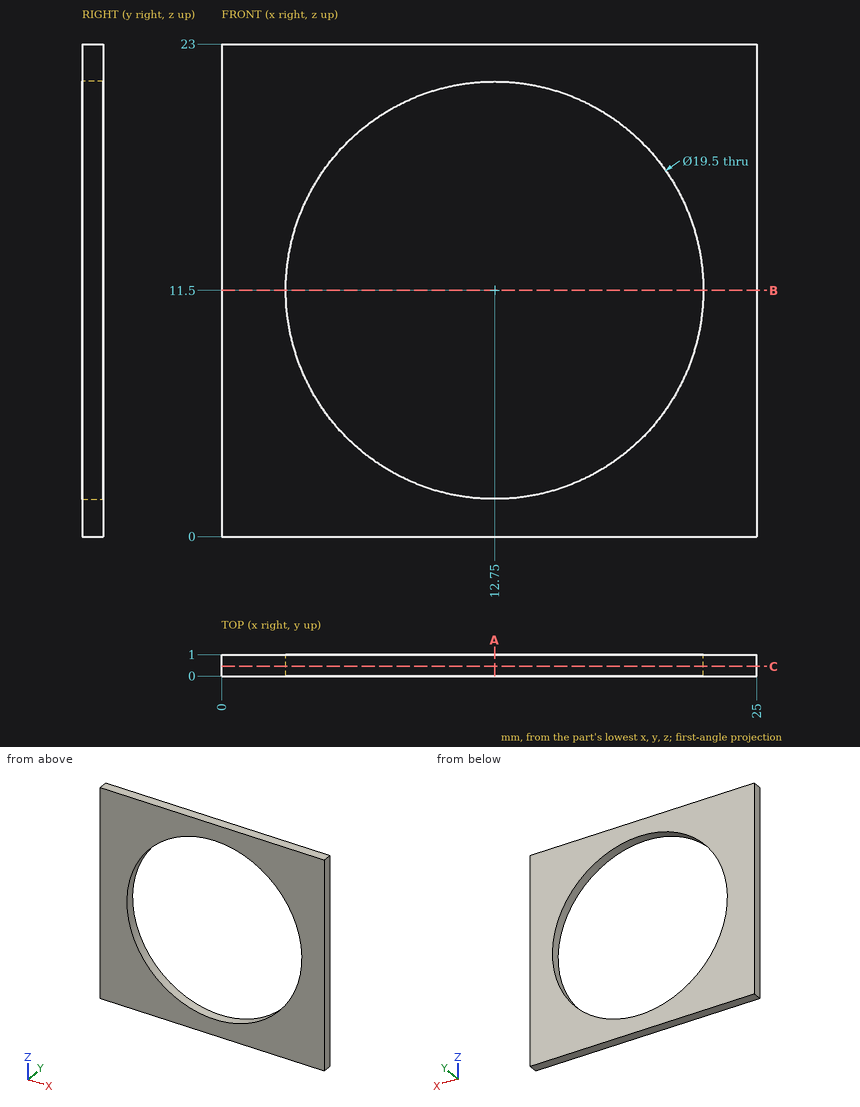
Study the drawing (mm; zero at the part's minimum x, y, z) and answer. Give positions to 0.01 mm unless a question says otherwise; leave off trailing zeros. Order: outer loops, then holes, each group sorted by start corner. A loop starts at its lowest first (then second) coordinate and runs counter-clockwise, first axis right, second up.
1. Straight lines are drawn through the part: L1, parallel to X at y = 0.3, z = 11.5; L2, parallel to X at y = 0.45, z = 7.25; L3, parallel to Z at x = 17.25, y = 0.5. For each, find the intervals that lie inside material, in ascending order.
Result sheet:
L1: x = 0 to 3, 22.5 to 25
L2: x = 0 to 3.98, 21.52 to 25
L3: z = 0 to 2.85, 20.15 to 23
2. Section B-B, the plane z = 11.5 is taken. Determine the outline of the cut face in (x, y).
Result sheet:
outline: (0, 0) - (3, 0) - (3, 1) - (0, 1) - close; (22.5, 0) - (25, 0) - (25, 1) - (22.5, 1) - close
3. Section A-A, the plane x = 12.75 is taken. Determine the outline of the cut face in (y, z), and give its area (3 significant figures).
Result sheet:
outline: (0, 0) - (1, 0) - (1, 1.75) - (0, 1.75) - close; (0, 21.25) - (1, 21.25) - (1, 23) - (0, 23) - close
area: 3.50 mm2
4. Section C-C, the plane y = 0.45 is taken. Determine the outline of the cut face in (x, z), and give its area (3 significant figures).
Result sheet:
outline: (0, 0) - (25, 0) - (25, 23) - (0, 23) - close; hole circle Ø19.5 at (12.75, 11.5)
area: 276 mm2
